Source: CAD feature listing. Evaluate the final solid. Frame: model axes, mm. Face numbers are marked on the shaded views. A direction names the side the tool comes from. Coordinates: 2 decimals unless noted, no trailing zeros. Order: outer loops, then holes, each group sorted by start corner. A loop starts at its lowest first (then second) coordinate and runs counter-clockwise, first axis right, second up.
Item 1: Section A-A on x = 32. Return the cut outline in (y, z), then the cut area to 3 significant figures.
Item 2: Contact query for a flat-ended pin moving along its axis: P1, Ø1.5, axis at x = 13.5, y = 13.5, coming from the +Z side. Output: stop coordinate, or through.
Item 3: Section B-B on z = 7.75. Return the cut outline in (x, y).
Item 4: Mould query, pull axis Y, two halves, no side actions, for the marked faces 3, 4, 5 and 6. Classes: released by +Y, released by -Y, zero draft, split by the parting line, or undercut.
Item 5: Ray query, line 1 (X direction, y = 22, z = 5.75); line 2 (X direction, y = 51, z = 4.7); line 3 (Y direction, x = 28, z = 8). Return the intervals inside material, ascending.
Item 6: Section C-C on x = 13. Return the cut outline in (y, z), then the cut area to 3 significant figures.
Item 7: Reachability of the marked faces 1 and 2 from +Z, -Z, +X, -X, +Y, -Y: full face, straight path, thin tool, end or side. Return the list, or none.
Item 8: Section D-D on y = 24.5. Return the cut outline in (x, z), then the cut area to 3 significant figures.
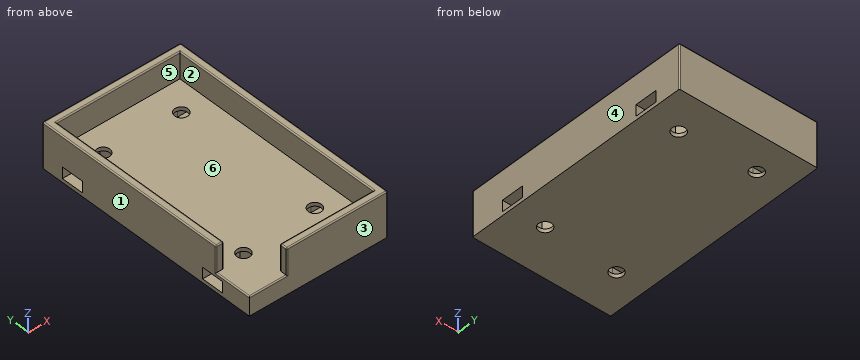
from build123d import *

# Parameters (mm, degrees)
PRISM003_DEPTH            = 3
CYLINDER005_R             = 1.75
CYLINDER005_DEPTH         = 20
BOX004_W                  = 6
BOX004_H                  = 20
BOX004_DEPTH              = 3
FUSION001_PLACEMENT_ANGLE = 90
PRISM004_DEPTH            = 3
CYLINDER006_R             = 1.75
CYLINDER006_DEPTH         = 20
BOX005_W                  = 6
BOX005_H                  = 20
BOX005_DEPTH              = 3
FUSION002_PLACEMENT_ANGLE = 270
PRISM005_DEPTH            = 3
CYLINDER007_R             = 1.75
CYLINDER007_DEPTH         = 20
BOX006_W                  = 6
BOX006_H                  = 20
BOX006_DEPTH              = 3
FUSION003_PLACEMENT_ANGLE = 90
PRISM002_DEPTH            = 3
CYLINDER004_R             = 1.75
CYLINDER004_DEPTH         = 20
BOX003_W                  = 6
BOX003_H                  = 20
BOX003_DEPTH              = 3
FUSION_PLACEMENT_ANGLE    = 90
BOX002_W                  = 10
BOX002_H                  = 10
BOX002_DEPTH              = 10
BOX_W                     = 33
BOX_H                     = 58
BOX_DEPTH                 = 10
BOX001_W                  = 37
BOX001_H                  = 62
BOX001_DEPTH              = 12
FILLET_R                  = 0.3
FILLET001_R               = 0.3


with BuildPart() as prisma003:
    # Prism003 → Prism003 (new body)
    with BuildSketch(Plane(origin=(34, 7.5, 3), x_dir=(0, 1, 0), z_dir=(0, 0, 1))):
        Polygon((3.25, 0), (1.625, 2.814583), (-1.625, 2.814583), (-3.25, 0), (-1.625, -2.814583), (1.625, -2.814583), align=None)
    extrude(amount=PRISM003_DEPTH)


with BuildPart() as cilindro005:
    # Cylinder005 → Cylinder005 (new body)
    with BuildSketch(Plane(origin=(34, 7.5, -1), x_dir=(1, 0, 0), z_dir=(0, 0, 1))):
        Circle(CYLINDER005_R)
    extrude(amount=CYLINDER005_DEPTH)


with BuildPart() as fusion001:
    # Box004 → Box004 (new body)
    with BuildSketch(Plane(origin=(31, 9, 3), x_dir=(1, 0, 0), z_dir=(0, 0, 1))):
        with Locations((3, 10)):
            Rectangle(BOX004_W, BOX004_H)
    extrude(amount=BOX004_DEPTH)

    # Fusion001: union Prisma003, Cilindro005
    add(prisma003.part)
    add(cilindro005.part)


with BuildPart() as fusion001_1:
    # Fusion001 placement: moved
    add(fusion001.part.moved(Location((13.75, -25, -2))).rotate(Axis((13.75, -25, -2), (0, 0, 1)), FUSION001_PLACEMENT_ANGLE))


with BuildPart() as prisma004:
    # Prism004 → Prism004 (new body)
    with BuildSketch(Plane(origin=(34, 7.5, 3), x_dir=(0, 1, 0), z_dir=(0, 0, 1))):
        Polygon((3.25, 0), (1.625, 2.814583), (-1.625, 2.814583), (-3.25, 0), (-1.625, -2.814583), (1.625, -2.814583), align=None)
    extrude(amount=PRISM004_DEPTH)


with BuildPart() as cilindro006:
    # Cylinder006 → Cylinder006 (new body)
    with BuildSketch(Plane(origin=(34, 7.5, -1), x_dir=(1, 0, 0), z_dir=(0, 0, 1))):
        Circle(CYLINDER006_R)
    extrude(amount=CYLINDER006_DEPTH)


with BuildPart() as fusion002:
    # Box005 → Box005 (new body)
    with BuildSketch(Plane(origin=(31, 9, 3), x_dir=(1, 0, 0), z_dir=(0, 0, 1))):
        with Locations((3, 10)):
            Rectangle(BOX005_W, BOX005_H)
    extrude(amount=BOX005_DEPTH)

    # Fusion002: union Prisma004, Cilindro006
    add(prisma004.part)
    add(cilindro006.part)


with BuildPart() as fusion002_1:
    # Fusion002 placement: moved
    add(fusion002.part.moved(Location((18.75, 44, -2))).rotate(Axis((18.75, 44, -2), (0, 0, 1)), FUSION002_PLACEMENT_ANGLE))


with BuildPart() as prisma005:
    # Prism005 → Prism005 (new body)
    with BuildSketch(Plane(origin=(34, 7.5, 3), x_dir=(0, 1, 0), z_dir=(0, 0, 1))):
        Polygon((3.25, 0), (1.625, 2.814583), (-1.625, 2.814583), (-3.25, 0), (-1.625, -2.814583), (1.625, -2.814583), align=None)
    extrude(amount=PRISM005_DEPTH)


with BuildPart() as cilindro007:
    # Cylinder007 → Cylinder007 (new body)
    with BuildSketch(Plane(origin=(34, 7.5, -1), x_dir=(1, 0, 0), z_dir=(0, 0, 1))):
        Circle(CYLINDER007_R)
    extrude(amount=CYLINDER007_DEPTH)


with BuildPart() as fusion003:
    # Box006 → Box006 (new body)
    with BuildSketch(Plane(origin=(31, 9, 3), x_dir=(1, 0, 0), z_dir=(0, 0, 1))):
        with Locations((3, 10)):
            Rectangle(BOX006_W, BOX006_H)
    extrude(amount=BOX006_DEPTH)

    # Fusion003: union Prisma005, Cilindro007
    add(prisma005.part)
    add(cilindro007.part)


with BuildPart() as fusion003_1:
    # Fusion003 placement: moved
    add(fusion003.part.moved(Location((18.75, 84, -2))).rotate(Axis((18.75, 84, -2), (0, 0, -1)), FUSION003_PLACEMENT_ANGLE))


with BuildPart() as prisma002:
    # Prism002 → Prism002 (new body)
    with BuildSketch(Plane(origin=(34, 7.5, 3), x_dir=(0, 1, 0), z_dir=(0, 0, 1))):
        Polygon((3.25, 0), (1.625, 2.814583), (-1.625, 2.814583), (-3.25, 0), (-1.625, -2.814583), (1.625, -2.814583), align=None)
    extrude(amount=PRISM002_DEPTH)


with BuildPart() as cilindro004:
    # Cylinder004 → Cylinder004 (new body)
    with BuildSketch(Plane(origin=(34, 7.5, -1), x_dir=(1, 0, 0), z_dir=(0, 0, 1))):
        Circle(CYLINDER004_R)
    extrude(amount=CYLINDER004_DEPTH)


with BuildPart() as fusion004:
    # Box003 → Box003 (new body)
    with BuildSketch(Plane(origin=(31, 9, 3), x_dir=(1, 0, 0), z_dir=(0, 0, 1))):
        with Locations((3, 10)):
            Rectangle(BOX003_W, BOX003_H)
    extrude(amount=BOX003_DEPTH)

    # Fusion: union Prisma002, Cilindro004
    add(prisma002.part)
    add(cilindro004.part)


with BuildPart() as fusion004_1:
    # Fusion placement: moved
    add(fusion004.part.moved(Location((13.75, 17, -2))).rotate(Axis((13.75, 17, -2), (0, 0, 1)), FUSION_PLACEMENT_ANGLE))

    # Fusion004: union Fusion001, Fusion002, Fusion003
    add(fusion001_1.part)
    add(fusion002_1.part)
    add(fusion003_1.part)


with BuildPart() as cubo002:
    # Box002 → Box002 (new body)
    with BuildSketch(Plane(origin=(-2, -2, 5), x_dir=(1, 0, 0), z_dir=(0, 0, 1))):
        with Locations((5, 5)):
            Rectangle(BOX002_W, BOX002_H)
    extrude(amount=BOX002_DEPTH)


with BuildPart() as cubo:
    # Box → Box (new body)
    with BuildSketch(Plane.XY.offset(5)):
        with Locations((16.5, 29)):
            Rectangle(BOX_W, BOX_H)
    extrude(amount=BOX_DEPTH)


with BuildPart() as fillet001:
    # Box001 → Box001 (new body)
    with BuildSketch(Plane(origin=(-2, -2, 0), x_dir=(1, 0, 0), z_dir=(0, 0, 1))):
        with Locations((18.5, 31)):
            Rectangle(BOX001_W, BOX001_H)
    extrude(amount=BOX001_DEPTH)

    # Cut: cut Cubo
    add(cubo.part, mode=Mode.SUBTRACT)

    # Cut001: cut Cubo002
    add(cubo002.part, mode=Mode.SUBTRACT)

    # Cut002: cut Fusion004
    add(fusion004_1.part, mode=Mode.SUBTRACT)

    # Fillet
    fillet_edges = [fillet001.edges().sort_by_distance(p)[0] for p in [
        (-2, 60, 6),
        (-2, 34, 12),
        (35, -2, 6),
        (21.5, -2, 12),
        (35, 60, 6),
        (16.5, 60, 12),
        (35, 29, 12),
        (20.5, 0, 12),
        (33, 29, 12),
        (16.5, 58, 12),
        (0, 33, 12),
    ]]
    fillet(fillet_edges, radius=FILLET_R)

    # Fillet001
    fillet001_edges = [fillet001.edges().sort_by_distance(p)[0] for p in [
        (-2, 3, 5),
        (-2, 8, 8.35),
        (8, -2, 8.35),
        (3, -2, 5),
        (0, 8, 8.35),
        (-1, 8, 12),
        (8, 0, 8.35),
        (8, -1, 12),
    ]]
    fillet(fillet001_edges, radius=FILLET001_R)


solid = fillet001.part
Answer list:
1. outline: (-2, 0) - (60, 0) - (60, 11.7) arc R0.3 ccw to (59.7, 12) - (58.3, 12) arc R0.3 ccw to (58, 11.7) - (58, 5) - (0, 5) - (0, 11.7) arc R0.3 ccw to (-0.3, 12) - (-1.7, 12) arc R0.3 ccw to (-2, 11.7) - close; hole (7, 1) - (13, 1) - (13, 4) - (7, 4) - close; hole (47, 1) - (53, 1) - (53, 4) - (47, 4) - close
1. area: 302 mm2
2. P1: stops at z = 5
3. outline: (-2, 8.3) arc R0.3 ccw to (-1.7, 8) - (-0.3, 8) arc R0.3 ccw to (0, 8.3) - (0, 58) - (33, 58) - (33, 0) - (8.3, 0) arc R0.3 ccw to (8, -0.3) - (8, -1.7) arc R0.3 ccw to (8.3, -2) - (34.7, -2) arc R0.3 ccw to (35, -1.7) - (35, 59.7) arc R0.3 ccw to (34.7, 60) - (-1.7, 60) arc R0.3 ccw to (-2, 59.7) - close
4. face 3: released by -Y
4. face 4: zero draft
4. face 5: undercut
4. face 6: undercut
5. line 1: x = -2 to 0, 33 to 35
5. line 2: x = -2 to 4.5, 8 to 24.81, 27.69 to 35
5. line 3: y = -2 to 0, 58 to 60
6. outline: (-2, 0) - (60, 0) - (60, 11.7) arc R0.3 ccw to (59.7, 12) - (58.3, 12) arc R0.3 ccw to (58, 11.7) - (58, 5) - (0, 5) - (0, 11.7) arc R0.3 ccw to (-0.3, 12) - (-1.7, 12) arc R0.3 ccw to (-2, 11.7) - close
6. area: 338 mm2
7. face 1: +Z, -Z, -X, +Y, -Y
7. face 2: +Z
8. outline: (-2, 0) - (35, 0) - (35, 11.7) arc R0.3 ccw to (34.7, 12) - (33.3, 12) arc R0.3 ccw to (33, 11.7) - (33, 5) - (0, 5) - (0, 11.7) arc R0.3 ccw to (-0.3, 12) - (-1.7, 12) arc R0.3 ccw to (-2, 11.7) - close
8. area: 213 mm2
